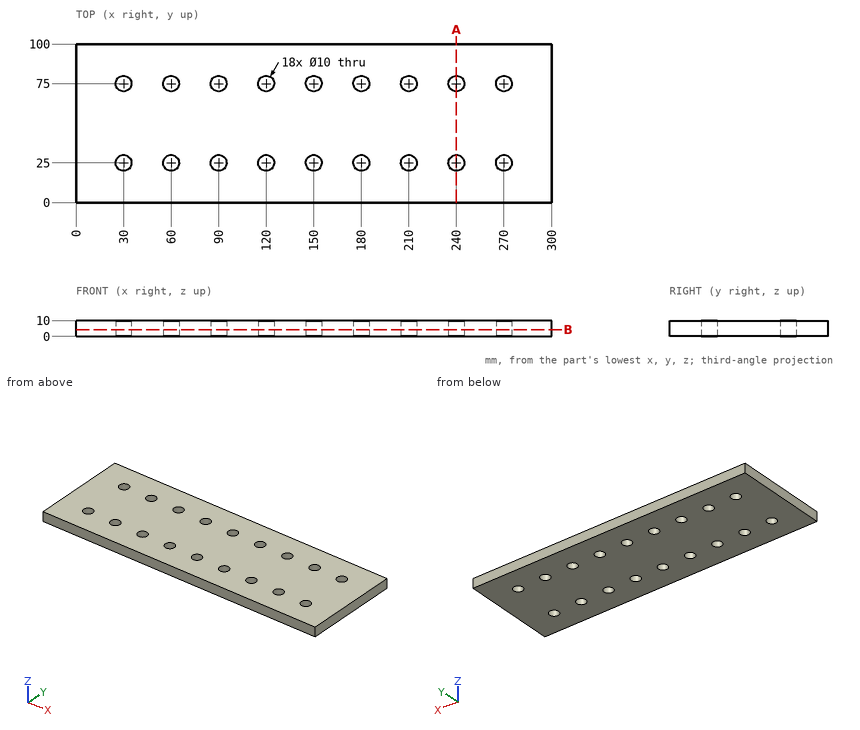
The drawing under review shows one solid part. Ordinate dimensions are in mm from its lowest x, y, z. Coordinates: 2 decimals unless noted, no trailing zeros. Loops run counter-clockwise (first coordinate to the right, second up) from the corner with the lowest first, then second, coordinate; pieces in that order, holes last. Notation, with made-up numbers: (37, 42) -> (54, 42) arc R30 cw to (54, 77) -> close; hole circle Ø9 at (53, 74.5). An arc over 180 degrees is marked (long way). Answer as a JSON object with one key per item and string values.
Q1. Clearance check with a flat-ended pin moving along its axis: pin 1 Ø5 at (x, y) = (153.5, 52) entering from -Z. State where the tip first meets the part, or that it passes through.
Answer block:
{"pin 1": "stops at z = 0"}
Q2. To check wall thickness, follow L1, parallel to Y at x = 120, z = 5.5; L2, parallel to Y at x = 31, z = 8.5. State the ranges of each line that lie inside material, in increasing order.
Answer block:
{"L1": "y = 0 to 20, 30 to 70, 80 to 100", "L2": "y = 0 to 20.1, 29.9 to 70.1, 79.9 to 100"}
Q3. Take a section at B-B on z = 4.25. Give the number of separate pieces and of enclosed holes in the cut face, plus the area to 3 significant figures.
Answer block:
{"separate pieces": "1", "enclosed holes": "18", "area": "28,600 mm^2"}
Q4. Take a section at A-A on x = 240. Give the boundary of the cut face in (y, z).
Answer block:
{"outline": "(0, 0) -> (20, 0) -> (20, 10) -> (0, 10) -> close; (30, 0) -> (70, 0) -> (70, 10) -> (30, 10) -> close; (80, 0) -> (100, 0) -> (100, 10) -> (80, 10) -> close"}
